from build123d import *

# Parameters (mm, degrees)
SKETCH1_W          = 22
SKETCH1_H          = 18.1
SKETCH2_R          = 3.71375
CUT_EXTRUDE1_DEPTH = 8.5725
SKETCH4_R          = 3.71375
CUT_EXTRUDE2_DEPTH = 8.5725


with BuildPart() as part:
    # Sketch1 → Revolve1 (revolve)
    with BuildSketch(Plane.XY):
        with Locations((19.255, 9.05)):
            Rectangle(SKETCH1_W, SKETCH1_H)
    revolve(axis=Axis((8.255, 0, 0), (1, 0, 0)))

    # Sketch2 → Cut-Extrude1 (cut)
    with BuildSketch(Plane.ZY.offset(-8.255)):
        Circle(SKETCH2_R)
    extrude(amount=-CUT_EXTRUDE1_DEPTH, mode=Mode.SUBTRACT)

    # Sketch4 → Cut-Extrude2 (cut)
    with BuildSketch(Plane(origin=(30.255, 0, 0), x_dir=(0, 0, -1), z_dir=(1, 0, 0))):
        Circle(SKETCH4_R)
    extrude(amount=-CUT_EXTRUDE2_DEPTH, mode=Mode.SUBTRACT)


solid = part.part
Geometry check sheet. Reference: the model listing, model coordinates, mm. A direction names the side the tool comes from. Give positions to 0.01 mm unless a question says otherwise; leave off trailing zeros. Write each loop counter-clockwise with the first axis right and the second up, starting at its lowest first coordinate (ties: lowest second). Pieces come first, ordered by that corner, then holes. Notation, with made-up numbers: M 65.5,23.5 L 121.5,23.5 A22 cw 121.5,53.5 Z; hole C 88,79.5 d11. An arc over 180 degrees is marked long. Answer as CSV lines item,"result". Start each with the question number.
Q1. Material ranges on L1, parallel to Z at x = 17.75, y = 0.5; L2, parallel to Z at x = 26.5, y = -1.5; L3, parallel to Z at x = 21.25, y = -5.5, recorded low to high.
Q2. Tool access check on faces 4 (the face through (21.682, 0, 0)), 5 (the face through (30.255, -4, 0)), 6 (the face through (12.481, -3.625, -0.805)). Record the directions out of +Z, -Z, +X, -X, +Y, -Y that give a thin tool (end or side, any length) a straight path to the whole face; none if there is none.
Q3. Section check C-C, the plane y = 2.5. Record the cut outline in (x, z) (1 decimal), then the cut area to 3 significant figures.
Q4. Go/stop test with flat-tipped pins: pin 1 (8 mm diameter, centred on x = 18, z = -14.5, fed in from +Y); pin 2 (2 mm diameter, centred on y = 0.5, z = 0, fed in from -X); pin 3 (6.5 mm diameter, centred on y = 0, z = 0, fed in from +X). Record where each tip stops, or that it passes through.
Q5. Section check D-D, the plane x = 19. Record the cut outline in (y, z).
Q6. Release check for a two-part mould opening along Y. For faces 1 (the face through (8.255, -4, 0)), 2 (the face through (19.409, 17.264, 5.437)), 3 (the face through (26.029, -3.625, 0.805)) record: pulls with the +Y half, pulls with the -Y half, needs draft (parallel to the pull), parting line crosses it, or undercut.
Q7. Section check A-A, the plane x = 12. Record the cut outline in (y, z).
Q8. Section check B-B, the plane z = -2. Record the cut outline in (x, y) (1 decimal).
Geometry says:
1,L1,"-18.09 to 18.09"
1,L2,"-18.04 to -3.4, 3.4 to 18.04"
1,L3,"-17.24 to 17.24"
2,face 4,"+X"
2,face 5,"+Z, -Z, +X, +Y, -Y"
2,face 6,"-X"
3,outline,"M 8.3,-17.9 L 30.3,-17.9 L 30.3,-2.7 L 21.7,-2.7 L 21.7,2.7 L 30.3,2.7 L 30.3,17.9 L 8.3,17.9 L 8.3,2.7 L 16.8,2.7 L 16.8,-2.7 L 8.3,-2.7 Z"
3,area,"695 mm^2"
4,pin 1,"y = 14.74"
4,pin 2,"x = 16.83"
4,pin 3,"x = 21.68"
5,outline,"C 0,0 d36.2"
6,face 1,"needs draft"
6,face 2,"parting line crosses it"
6,face 3,"undercut"
7,outline,"C 0,0 d36.2; hole C 0,0 d7.43"
8,outline,"M 8.3,-18 L 30.3,-18 L 30.3,-3.1 L 21.7,-3.1 L 21.7,3.1 L 30.3,3.1 L 30.3,18 L 8.3,18 L 8.3,3.1 L 16.8,3.1 L 16.8,-3.1 L 8.3,-3.1 Z"
